Job drawing, mm, ordinate dimensions from the low corner. One solid piece. A direction names the side the tool comes from. Give positions to 0.01 mm unless a question says otherwise; leave off trailing zeros. Loops run counter-clockwise (first coordinate to the right, second up) from the corner with the lowest first, then second, coordinate; pieces in that order, holes last. Notation, with made-up numbers: (75.25, 13.5) -> (129.25, 13.5) arc R37 ccw to (129.25, 49.5) -> close; hole circle Ø3 at (53.25, 44.25). An arc over 180 degrees is marked (long way). Answer as a JSON object with one key per item and string values. Group by question number.
Q1. Band-saw the part on B-B, the plane z = 4. Write the cut outline in (x, y).
Q2. Band-saw the part on C-C, the plane x = 13.25. Write the cut outline in (y, z), plus the area to 3 significant figures.
Q3. Band-saw the part on D-D, the plane y = 3.5. Write the cut outline in (x, z).
Q4. Two-plate mould, pull along Z, no slides. Class the marked faces 1, 2 and 3: pulls with the +Z half, pulls with the -Z half, needs draft (parallel to the pull), parting line crosses it, or undercut.
Q5. Band-saw the part on A-A, the plane x = 2.4. Write the cut outline in (y, z).
Q6. Drop a flat-ended pin along its axis: pin 1 (4.5 mm diameter, centred on x = 16.5, y = 12.6, fed in from +Z). Give the stop position or say it passes through.
Q7. Wall check: probe 1 along X at (y, z) = (12.5, 0.75); probe 2 along Y at (x, z) = (16.5, 0.35); probe 3 along Z at (x, y) = (14.75, 3.5). Give the ranges that are in metal, low to high. Write a range as from..to.
Q8. Tool access for the marked faces 4, 5, 6 and 7: list every direction of +Z, -Z, +X, -X, +Y, -Y with a clear straight run to the whole face (end or side of a thin tool).
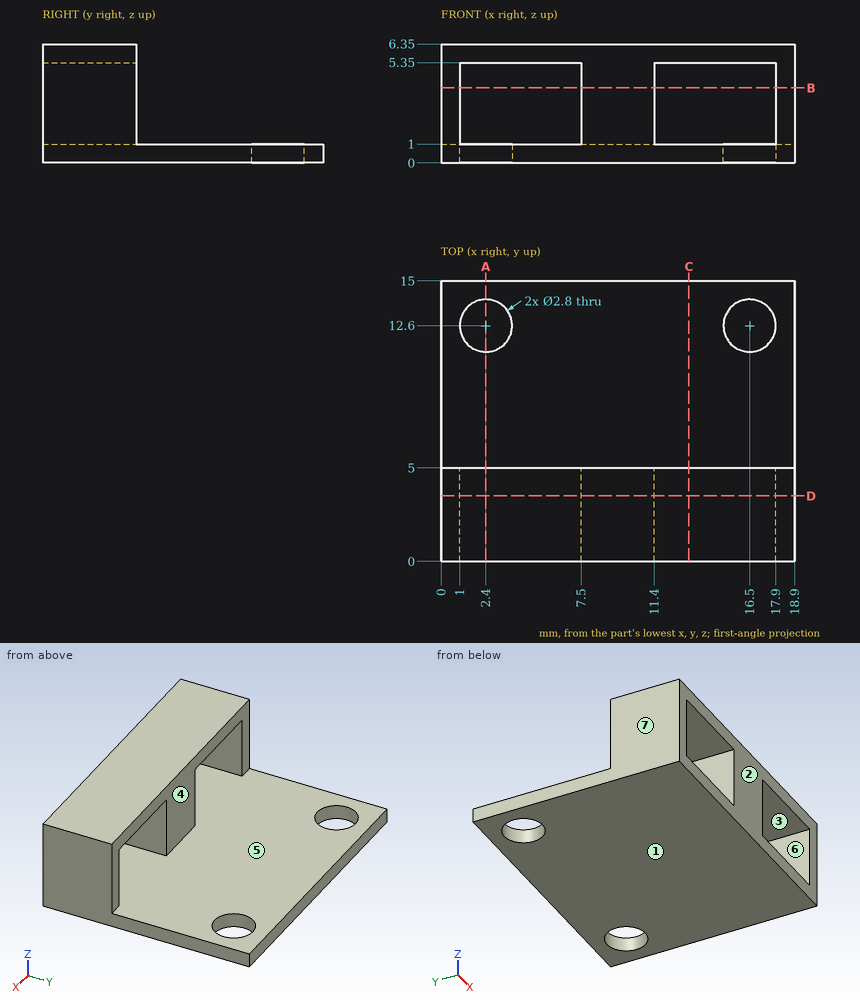
Worked answers:
{
 "1": {"outline": "(0, 0) -> (1, 0) -> (1, 5) -> (0, 5) -> close; (7.5, 0) -> (11.4, 0) -> (11.4, 5) -> (7.5, 5) -> close; (17.9, 0) -> (18.9, 0) -> (18.9, 5) -> (17.9, 5) -> close"},
 "2": {"outline": "(0, 0) -> (15, 0) -> (15, 1) -> (0, 1) -> close; (0, 5.35) -> (5, 5.35) -> (5, 6.35) -> (0, 6.35) -> close", "area": "20.0 mm2"},
 "3": {"outline": "(0, 0) -> (18.9, 0) -> (18.9, 6.35) -> (0, 6.35) -> close; hole (1, 1) -> (7.5, 1) -> (7.5, 5.35) -> (1, 5.35) -> close; hole (11.4, 1) -> (17.9, 1) -> (17.9, 5.35) -> (11.4, 5.35) -> close"},
 "4": {"face 1": "pulls with the -Z half", "face 2": "needs draft", "face 3": "undercut"},
 "5": {"outline": "(0, 0) -> (11.2, 0) -> (11.2, 1) -> (0, 1) -> close; (0, 5.35) -> (5, 5.35) -> (5, 6.35) -> (0, 6.35) -> close; (14, 0) -> (15, 0) -> (15, 1) -> (14, 1) -> close"},
 "6": {"pin 1": "z = 1"},
 "7": {"probe 1": "0..1, 3.8..15.1, 17.9..18.9", "probe 2": "0..11.2, 14..15", "probe 3": "0..1, 5.35..6.35"},
 "8": {"face 4": "+Z, +X, -X, +Y", "face 5": "+Y", "face 6": "+Y, -Y", "face 7": "+Z, -Z, -X, +Y, -Y"}
}
